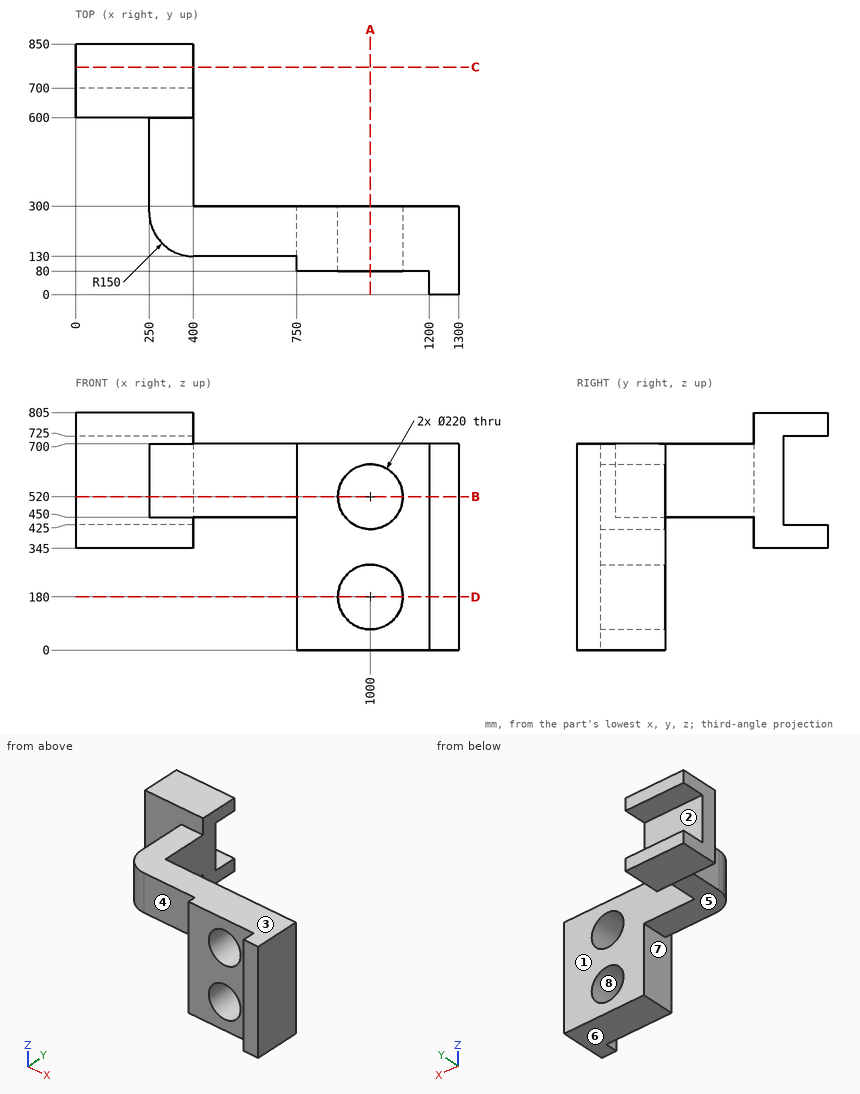
The figure shows three views and two pictorial views of one solid part (mm, origin at its lowest corner). Answer the questions. A direction names the side the tool comes from. Give positions to 0.01 mm unless a question says otherwise; leave off trailing zeros. Loops run counter-clockwise (first coordinate to the right, second up) from the corner with the lowest first, then second, coordinate; pieces in that order, holes last. Notation, with made-up numbers: (43.25, 25.25) - (102.25, 25.25) arc R19 ccw to (102.25, 31.25) - close; hole circle Ø2 at (36, 61). An arc over 180 degrees is marked (long way). Answer in a Markdown table with one row per item.
(1) A tool of negligible diameter and unlimited length cuts with its end or side. For the marked faces 1, 2, 3, 4 and 5, from which of +Z, -Z, +X, -X, +Y, -Y can it reach the whole face along a straight path? Write none if from no direction.
Results list:
| item | result |
|---|---|
| face 1 | +Z, -Z, +X, +Y |
| face 2 | +X, -X, +Y |
| face 3 | +Z, +X, -X, -Y |
| face 4 | +Z, -Z, -X, -Y |
| face 5 | -Z, -X, -Y |
(2) Flat-ended cylindrical pins translate along their axes: pin 1 Ø4 at (x, y) = (504, 235) entering from +Z; pin 2 Ø8 at (y, z) = (741.5, 356) entering from +X; pin 3 Ø5 at (x, z) = (542.5, 539) entering from +Y. Find the tip coordinate at first contact, or state that the pin passes through.
Results list:
| item | result |
|---|---|
| pin 1 | stops at z = 700 |
| pin 2 | stops at x = 400 |
| pin 3 | stops at y = 300 |
(3) Consider L1, parallel to Z at x = 1000, y = 212; L2, parallel to Z at x = 208, y = 794; L3, parallel to X at y = 256.5, z = 180. Determine where each line is inside the solid, lowest interval first. Write a range as [from, to].
Results list:
| item | result |
|---|---|
| L1 | z = [0, 70], [290, 410], [630, 700] |
| L2 | z = [345, 425], [725, 805] |
| L3 | x = [750, 890], [1110, 1300] |
(4) Section C-C (y = 771.5) is taken. Give the vertices of the cut face in (x, z), and give its area (3 significant figures).
Results list:
| item | result |
|---|---|
| outline | (0, 345) - (400, 345) - (400, 425) - (0, 425) - close; (0, 725) - (400, 725) - (400, 805) - (0, 805) - close |
| area | 64,000 mm² |
(5) Section A-A (x = 1000) is taken. Give the vertices of the cut face in (y, z).
Results list:
| item | result |
|---|---|
| outline | (80, 0) - (300, 0) - (300, 70) - (80, 70) - close; (80, 290) - (300, 290) - (300, 410) - (80, 410) - close; (80, 630) - (300, 630) - (300, 700) - (80, 700) - close |
(6) Section D-D (z = 180) is taken. Give the vertices of the cut face in (x, y).
Results list:
| item | result |
|---|---|
| outline | (750, 80) - (890, 80) - (890, 300) - (750, 300) - close; (1110, 80) - (1200, 80) - (1200, 0) - (1300, 0) - (1300, 300) - (1110, 300) - close |
(7) For a pull along Z with two mould halves and no side action, classify the marked faces 6, 7 and 8 as pulls with the +Z half, pulls with the -Z half, needs draft (parallel to the pull), parting line crosses it, or undercut.
Results list:
| item | result |
|---|---|
| face 6 | pulls with the -Z half |
| face 7 | needs draft |
| face 8 | undercut |
(8) Section B-B (z = 520) is taken. Give the vertices of the cut face in (x, y).
Results list:
| item | result |
|---|---|
| outline | (0, 600) - (250, 600) - (250, 280) arc R150 ccw to (400, 130) - (750, 130) - (750, 80) - (890, 80) - (890, 300) - (400, 300) - (400, 700) - (0, 700) - close; (1110, 80) - (1200, 80) - (1200, 0) - (1300, 0) - (1300, 300) - (1110, 300) - close |
